Could you check a few things on this drawing? It's one solid part, dimensions in mm from its lowest x, y, z. Round coordinates to 2 decimals unless told otherwise and drop trailing zeros. Loops run counter-clockwise (first coordinate to the right, second up) from the corner with the lowest first, then second, coordinate; pieces in that order, holes last. Notation, with made-up numbers: (-16.75, 27.25) -> (0.25, 27.25) arc R23 ccw to (0.25, 49.25) -> close; hole circle Ø11 at (53, 64.25). An arc over 180 degrees is marked (long way). Write each question's results on one line, items separated by ' | '.
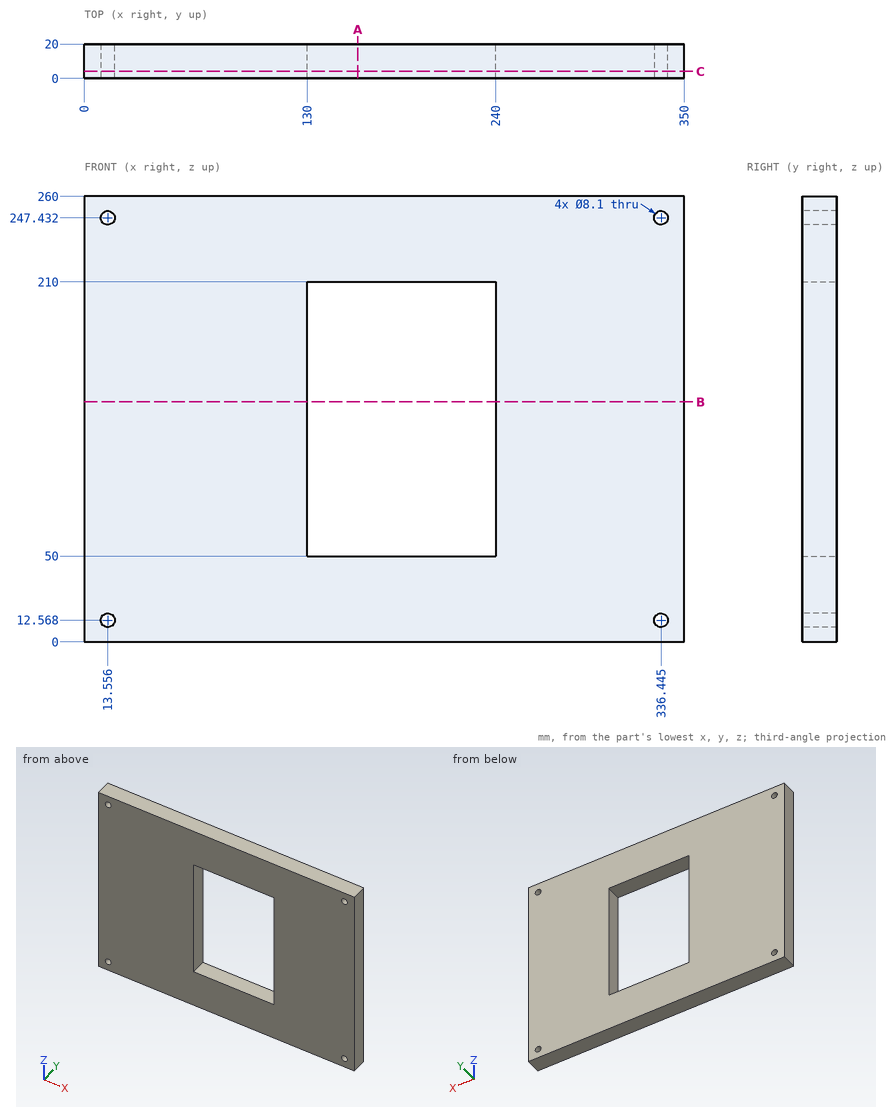
1) I want a section at B-B, the plane z = 140. Write out the boundary of the cut face in (x, y), plus the area to 3 significant figures.
Model answer:
outline: (0, 0) -> (130, 0) -> (130, 20) -> (0, 20) -> close; (240, 0) -> (350, 0) -> (350, 20) -> (240, 20) -> close | area: 4,800 mm2
2) I want a section at C-C, the plane y = 4. Give the number of separate pieces and of enclosed holes in the cut face, plus the area to 3 significant figures.
Model answer:
separate pieces: 1 | enclosed holes: 5 | area: 73,200 mm2
3) I need wall thicknesses on line 1 (Z direction, x = 218, y = 15.5); line 2 (X direction, y = 1, z = 59); line 3 (X direction, y = 2.25, z = 16) (1 decimal). Which ranges of each line are inside material? Lowest first, please.
Model answer:
line 1: z = 0 to 50, 210 to 260 | line 2: x = 0 to 130, 240 to 350 | line 3: x = 0 to 11.4, 15.7 to 334.3, 338.6 to 350
4) I want a section at A-A, the plane x = 159.5. Write out the boundary of the cut face in (y, z).
Model answer:
outline: (0, 0) -> (20, 0) -> (20, 50) -> (0, 50) -> close; (0, 210) -> (20, 210) -> (20, 260) -> (0, 260) -> close
